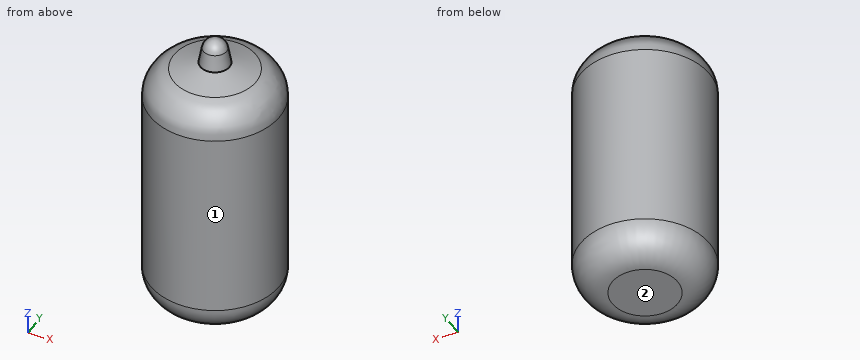
from build123d import *

# Parameters (mm, degrees)
F3_R = 5.08


with BuildPart() as f2:
    # F1 (on Front) → F2 (revolve)
    with BuildSketch(Plane.XZ):
        with BuildLine():
            Line((0, 0), (10.31875, 0))
            Line((10.31875, 0), (10.31875, 39.6875))
            Line((10.31875, 39.6875), (2.329721, 41.828154))
            Line((2.329721, 41.828154), (1.863166, 44.474118))
            ThreePointArc((1.863166, 44.474118), (1.216096, 45.594877), (0, 46.0375))
            Line((0, 46.0375), (0, 0))
        make_face()
    revolve(axis=Axis((0, 0, 23.01875), (0, 0, -1)))

    # F3
    f3_edges = [f2.edges().sort_by_distance(p)[0] for p in [
        (-10.31875, 0, 39.6875),
        (-10.31875, 0, 0),
    ]]
    fillet(f3_edges, radius=F3_R)


solid = f2.part
Geometry: final body of the model. Coordinates: model frame, mm. Face numbers are marked on the shaded views. Give positions to 0.01 mm unless a question says otherwise; leave off trailing zeros. Write each loop counter-clockwise with the first axis right and the second up, starting at its lowest first coordinate (ties: lowest second). Pieces come first, ordered by that corner, then holes.
(1) Ray query, line 1 (Z direction, x = 1, y = 5.25); line 2 (Y direction, x = 1.75, z = 27.5); line 3 (X direction, y = 5, z = 34). Return the intervals inside material, ascending.
(2) Mould query, pull axis X, two halves, no side actions, for the marked faces 1 and 2. Classes: released by +X, released by -X, zero draft, split by the parting line, or undercut.
(3) Cut plane A-A, the plane z = 14. Return loops of the section in (x, y), then the cut area to 3 significant figures.
(4) First-contact query: P1, Ø1.5, axis at x = -7, z = 21.5, coming from the -Y side; P2, Ø4, axis at y = 2.5, z = 17.5, coming from the +X side; P3, Ø3, axis at y = -5, z = 38.5, coming from the -X side. Flat tips, straight axial feed; report the tip coordinate or a pass-through.
Values follow:
1. line 1: z = 0 to 41.02
1. line 2: y = -10.17 to 10.17
1. line 3: x = -9.03 to 9.03
2. face 1: split by the parting line
2. face 2: zero draft
3. outline: circle Ø20.64 at (0, 0)
3. area: 335 mm2
4. P1: stops at y = -8.21
4. P2: stops at x = 10.31
4. P3: stops at x = -9.24
